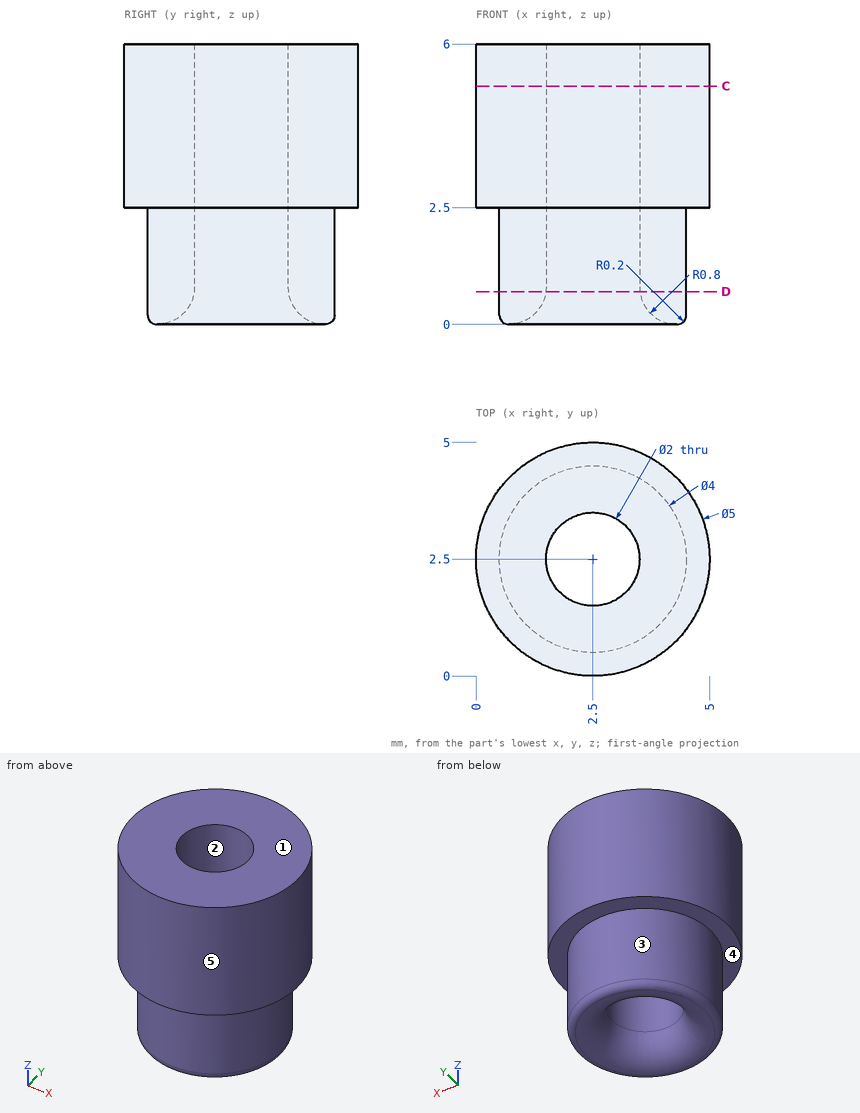
Can you work these out from the drawing? Everything is in mm from the part's minimum corner. A direction names the side the tool comes from. Give positions to 0.01 mm unless a question says otherwise; leave off trailing zeros. Write each loop counter-clockwise with the first axis right and the second up, starting at its lowest first coordinate (ties: lowest second). Pieces come first, ordered by that corner, then holes. Notation, with made-up numbers: (51.25, 10) -> (71.25, 10) arc R11 cw to (71.25, 21) -> close; hole circle Ø1 at (5.25, 38). An arc over 180 degrees is marked (long way). Write each question's results on one line, items separated by ' | '.
Item 1: Suppose I cut it at C-C on z = 5.1. Write out the boundary of the cut face in (x, y), plus the area to 3 significant figures.
Output:
outline: circle Ø5 at (2.5, 2.5); hole circle Ø2 at (2.5, 2.5) | area: 16.5 mm^2
Item 2: For pin 1 Ø2 at (y, z) = (1, 5) entering from -X; pin 2 Ø1 at (y, z) = (1.5, 4) entering from +X, each with a flat end and sliding along its axis, tell me the tip position at first contact or that it passes through.
Output:
pin 1: stops at x = 0.05 | pin 2: stops at x = 4.95
Item 3: If I drill on L1, parallel to Y at x = 2.5, z = 4.3; L2, parallel to Z at x = 0.4, y = 1.35; L3, parallel to X at y = 2.3, z = 4.7, over which ranges is the centre line in solid material (lowest first)?
Output:
L1: y = 0 to 1.5, 3.5 to 5 | L2: z = 2.5 to 6 | L3: x = 0.01 to 1.52, 3.48 to 4.99
Item 4: We'd pull the mould along Y, two halves only. Please class the marked faces 1, 2 and 3: pulls with the +Y half, pulls with the -Y half, needs draft (parallel to the pull), parting line crosses it, or undercut.
Output:
face 1: needs draft | face 2: undercut | face 3: parting line crosses it
Item 5: On a 3-axis mill with a long thin cutter (end or side, diameter ignored), from which of +Z, -Z, +X, -X, +Y, -Y can I reach the whole of each face in a straight line? I mean the marked faces 4 and 5. Say none if no direction works.
Output:
face 4: -Z | face 5: +Z, -Z
Item 6: Suppose I cut it at D-D on z = 0.7. Write out the boundary of the cut face in (x, y).
Output:
outline: circle Ø4 at (2.5, 2.5); hole circle Ø2.01 at (2.5, 2.5)
